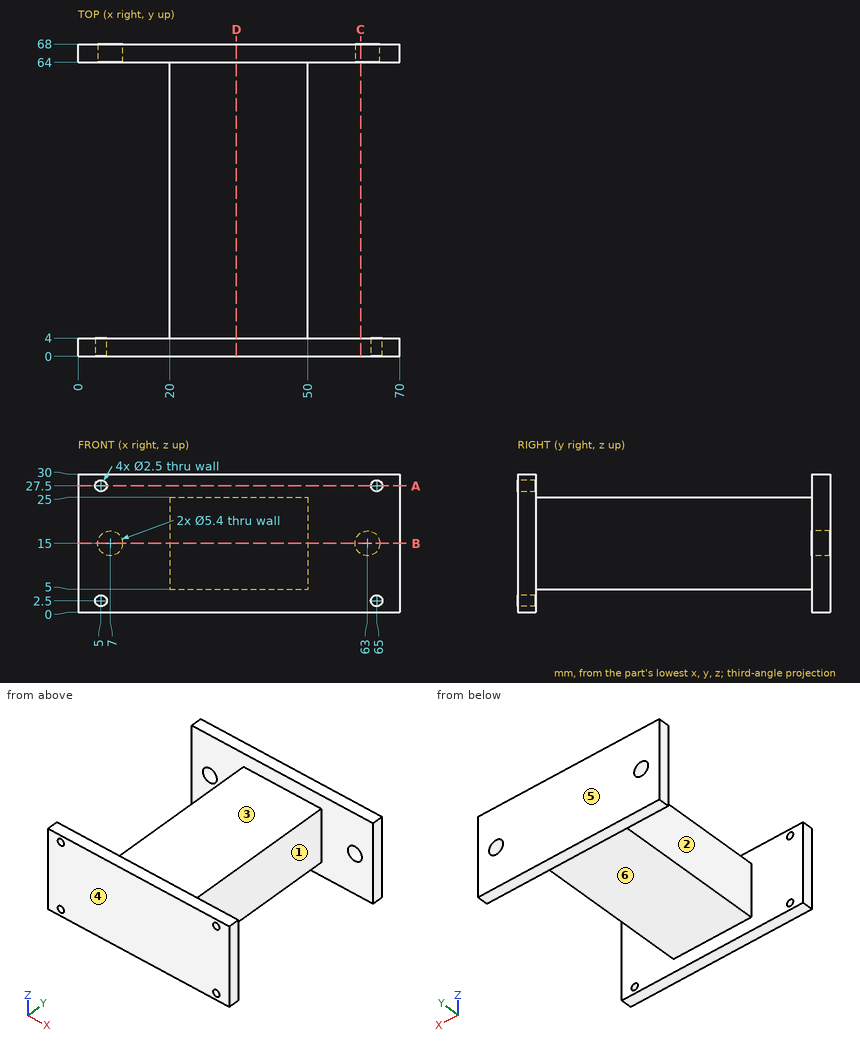
Could you check a few things on this drawing? It's one solid part, dimensions in mm from its lowest x, y, z. A direction names the side the tool comes from. Give positions to 0.01 mm unless a question says otherwise; leave off trailing zeros. Write each loop counter-clockwise with the first axis right and the second up, starting at its lowest first coordinate (ties: lowest second). Pieces come first, ordered by that corner, then holes. Notation, with made-up numbers: (30, 60.5) -> (34, 60.5) arc R14 ccw to (34, 79.5) -> close; hole circle Ø7 at (0, 15.25). An arc over 180 degrees is marked (long way). Answer as a JSON object with one key per item and string values.
Q1. Suppose I cut it at C-C on x = 61.5. Write out the boundary of the cut face in (y, z) (3 decimals), then the cut area to 3 significant figures.
Taken from the geometry:
{"outline": "(0, 0) -> (4, 0) -> (4, 30) -> (0, 30) -> close; (64, 0) -> (68, 0) -> (68, 12.755) -> (64, 12.755) -> close; (64, 17.245) -> (68, 17.245) -> (68, 30) -> (64, 30) -> close", "area": "222 mm²"}
Q2. Will these pins go through, and if not, where does the flat tip stop? pin 1 Ø16 at (y, z) = (29, 18) entering from +X; pin 2 Ø10 at (x, y) = (59, 15.5) entering from -Z; pin 3 Ø6 at (x, z) = (63, 15) entering from +Y; pin 4 Ø24 at (x, y) = (37, 42.5) entering from +Z.
Taken from the geometry:
{"pin 1": "stops at x = 50", "pin 2": "passes through", "pin 3": "stops at y = 68", "pin 4": "stops at z = 25"}
Q3. Suppose I cut it at B-B on z = 15. Write out the boundary of the cut face in (x, y).
Taken from the geometry:
{"outline": "(0, 0) -> (70, 0) -> (70, 4) -> (50, 4) -> (50, 64) -> (60.3, 64) -> (60.3, 68) -> (9.7, 68) -> (9.7, 64) -> (20, 64) -> (20, 4) -> (0, 4) -> close; (0, 64) -> (4.3, 64) -> (4.3, 68) -> (0, 68) -> close; (65.7, 64) -> (70, 64) -> (70, 68) -> (65.7, 68) -> close"}
Q4. Which directions (+Z, -Z, +X, -X, +Y, -Y) give clear straight access to the entire face, cutting with the end or side of a thin tool? Please do the marked faces 1, 2 and 3.
Taken from the geometry:
{"face 1": "+Z, -Z, +X", "face 2": "+Z, -Z, -X", "face 3": "+Z, +X, -X"}
Q5. Suppose I cut it at D-D on x = 34.5. Write out the boundary of the cut face in (y, z), then the cut area to 3 significant figures.
Taken from the geometry:
{"outline": "(0, 0) -> (4, 0) -> (4, 5) -> (64, 5) -> (64, 0) -> (68, 0) -> (68, 30) -> (64, 30) -> (64, 25) -> (4, 25) -> (4, 30) -> (0, 30) -> close", "area": "1,440 mm²"}
Q6. We'd pull the mould along Y, two halves only. Please class the marked faces 4, 5 and 6: released by +Y, released by -Y, zero draft, split by the parting line, or undercut.
Taken from the geometry:
{"face 4": "released by -Y", "face 5": "released by +Y", "face 6": "undercut"}
Q7. Please list where these lines run through material, in increasing order: L1, parallel to Z at x = 5, y = 1.35; L2, parallel to X at y = 2.5, z = 27.5; L3, parallel to X at y = 67.05, z = 15.
Taken from the geometry:
{"L1": "z = 0 to 1.25, 3.75 to 26.25, 28.75 to 30", "L2": "x = 0 to 3.75, 6.25 to 63.75, 66.25 to 70", "L3": "x = 0 to 4.3, 9.7 to 60.3, 65.7 to 70"}
Q8. Suppose I cut it at A-A on z = 27.5. Write out the boundary of the cut face in (x, y), then the cut area to 3 significant figures.
Taken from the geometry:
{"outline": "(0, 0) -> (3.75, 0) -> (3.75, 4) -> (0, 4) -> close; (0, 64) -> (70, 64) -> (70, 68) -> (0, 68) -> close; (6.25, 0) -> (63.75, 0) -> (63.75, 4) -> (6.25, 4) -> close; (66.25, 0) -> (70, 0) -> (70, 4) -> (66.25, 4) -> close", "area": "540 mm²"}
